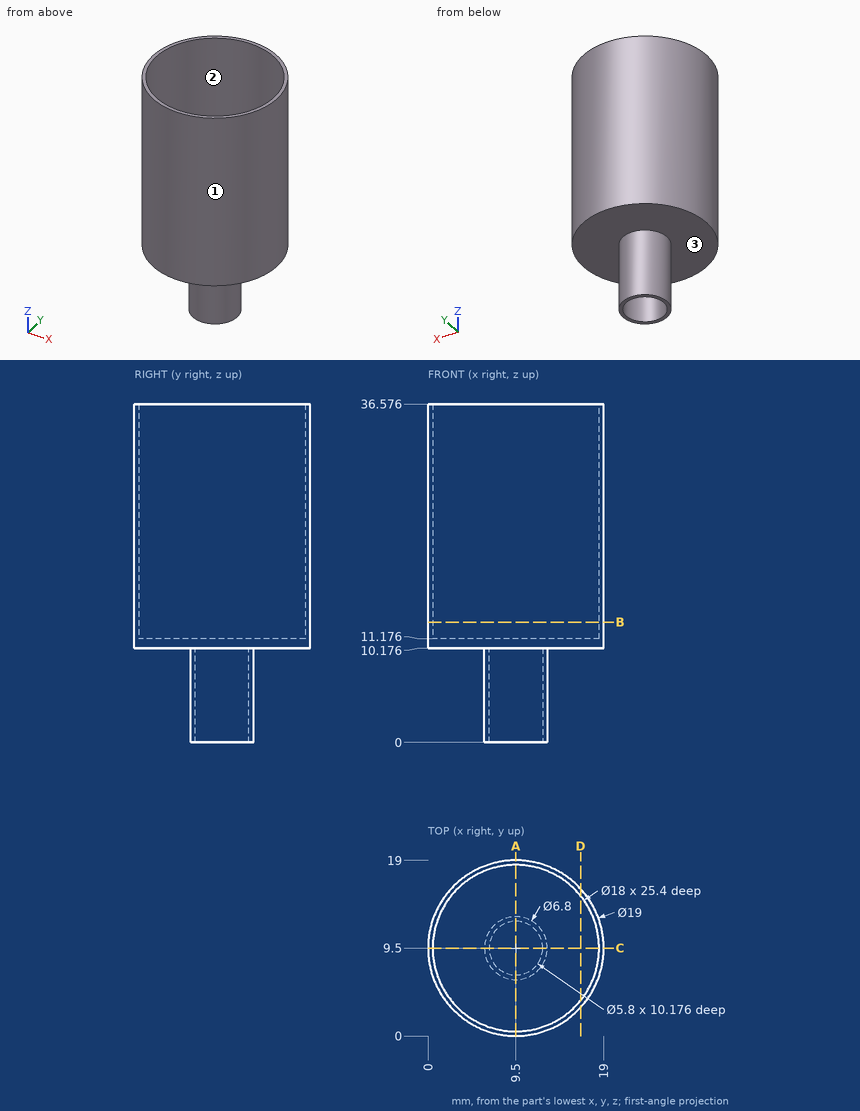
Job drawing, mm, ordinate dimensions from the low corner. One solid piece. Give positions to 0.01 mm unless a question says otherwise; leave off trailing zeros. Write each loop counter-clockwise with the first axis right and the second up, starting at its lowest first coordinate (ties: lowest second). Pieces come first, ordered by that corner, then holes. Notation, with made-up numbers: (2.25, 63) - (13.25, 63) arc R18 ccw to (13.25, 78) - close; hole circle Ø5 at (58.5, 85). An arc over 180 degrees is marked (long way). Answer as CSV lines item,"result".
1. Band-saw the part on B-B (z = 13). Write the cut outline in (x, y).
Responses:
outline,"circle Ø19 at (9.5, 9.5); hole circle Ø18 at (9.5, 9.5)"
2. Two-plate mould, pull along Y, no slides. Class the marked faces 1, 2 and 3: +Y half, -Y half, draft (parallel to the pull), parting line (faces both ways), or undercut.
Responses:
face 1,"parting line"
face 2,"undercut"
face 3,"draft"
3. Pin check, flat tips, straight feed: pin 1 (9 mm diameter, centred on x = 6, y = 11, fed in from +Z); pin 2 (5 mm diameter, centred on x = 3.5, z = 30.5, fed in from +Y); pin 3 (4 mm diameter, centred on x = 15, z = 4, fed in from +Y); pin 4 (4 mm diameter, centred on y = 7, z = 30, fed in from -X). Stop position of each tip, or through.
Responses:
pin 1,"stops at z = 11.18"
pin 2,"stops at y = 18.33"
pin 3,"passes through"
pin 4,"stops at x = 0.01"
4. Band-saw the part on A-A (x = 9.5). Write the cut outline in (y, z).
Responses:
outline,"(0, 10.18) - (6.1, 10.18) - (6.1, 0) - (6.6, 0) - (6.6, 10.18) - (12.4, 10.18) - (12.4, 0) - (12.9, 0) - (12.9, 10.18) - (19, 10.18) - (19, 36.58) - (18.5, 36.58) - (18.5, 11.18) - (0.5, 11.18) - (0.5, 36.58) - (0, 36.58) - close"
5. Band-saw the part on D-D (x = 16.5). Write the cut outline in (y, z).
Responses:
outline,"(3.08, 10.18) - (15.92, 10.18) - (15.92, 36.58) - (15.16, 36.58) - (15.16, 11.18) - (3.84, 11.18) - (3.84, 36.58) - (3.08, 36.58) - close"
6. Drill centre lines: L1, parallel to Y at x = 9.5, z = 23.25; L2, parallel to Y at x = 9.5, z = 5.25; L3, parallel to Z at x = 5.5, y = 1.5. Where is each one in solid material? Low to high. Write a range as [from, to].
Responses:
L1,"y = [0, 0.5], [18.5, 19]"
L2,"y = [6.1, 6.6], [12.4, 12.9]"
L3,"z = [10.18, 11.18]"
